The model under review builds one solid part; all positions refer to its coordinate system, in mm. A direction names the side the tool comes from. Coordinates: 2 decimals unless noted, no trailing zeros. Write each loop counter-clockwise with the first axis right and the second up, starting at its lowest first coordinate (ties: lowest second). Pieces come first, ordered by that corner, then holes.
Autodesk Inventor part; units mm, degrees
ref_plane "YZ Plane" through (0, 0, 0) normal (1, 0, 0) x (0, 1, 0)
ref_plane "XZ Plane" through (0, 0, 0) normal (0, 1, 0) x (-1, 0, 0)
ref_plane "XY Plane" through (0, 0, 0) normal (0, 0, 1) x (1, 0, 0)
sketch "Sketch1" plane through (0, 0, 0) normal (0, 0, 1) x (1, 0, 0)
  arc A0 (8.5146, 0.7768) -> (-8.5146, 0.7768) centre (0, 0) ccw
  line L0 (-18.6378, -8.55) -> (-30, -8.55)
  line L1 (30, -8.55) -> (30, -5.55)
  line L2 (30, -5.55) -> (17.1, -5.55)
  line L3 (-30, -8.55) -> (-30, -5.55)
  line L4 (-30, -5.55) -> (-17.1, -5.55)
  arc A1 (11.55, 0) -> (17.1, -5.55) centre (19.2544, 2.1544) ccw
  line L5 (11.55, 0) -> (17.1, -5.55) construction
  line L6 (11.55, 0) -> (19.3989, 0) construction
  arc A2 (8.4438, 1.3433) -> (18.6378, -8.55) centre (19.3906, 2.4242) ccw
  arc A3 (-17.1, -5.55) -> (-11.55, 0) centre (-19.2544, 2.1544) ccw
  arc A4 (-18.6378, -8.55) -> (-8.4438, 1.3433) centre (-19.3906, 2.4242) ccw
  line L7 (18.6378, -8.55) -> (30, -8.55)
  arc A5 (11.55, 0) -> (-11.55, 0) centre (0, 0) ccw
  dimension "d0" = 17.1
  dimension "d3" = 3
  dimension "d6" = 45
  dimension "d7" = 8
  dimension "d8" = 11
extrude "Extrusion1" add sketch "Sketch1" against normal blind 10 contours A0 A4 L0 L3 L4 A3 A5 A1 L2 L1 L7 A2
sketch "Sketch2" plane through (17.1, -5.55, 0) normal (0, 1, 0) x (1, 0, 0)
  circle A0 centre (6.45, 5) radius 1.5
  point P0 (-17.1, 0)
  dimension "d11" = 3
hole "Hole1" at (23.55, -5.55, -5) direction (0, -1, 0) diameter 3 end through all
sketch "Sketch3" plane through (-30, -5.55, 0) normal (0, 1, 0) x (1, 0, 0)
  circle A0 centre (6.45, 5) radius 1.5
  point P0 (30, 0)
  dimension "d19" = 3
hole "Hole2" at (-23.55, -5.55, -5) direction (0, -1, 0) diameter 3 end through all
sketch "Sketch4" plane through (-30, -8.55, 0) normal (0, -1, 0) x (1, 0, 0)
  circle A0 centre (6.45, -5) radius 1.5
  line L0 (0, -10) -> (11.3622, -10)
  line L1 (11.3622, 0) -> (11.3622, -10)
  line L2 (0, 0) -> (11.3622, 0)
  line L3 (0, 0) -> (0, -10)
  point P0 (30, 0)
properties part number "braket motor kipas"
Item 1: Take a section at A-A, the plane y = -4.75. Write out the cut boundary in (x, z).
Solved:
outline: (-15.21, -10) - (-11.05, -10) - (-11.05, 0) - (-15.21, 0) - close; (11.05, -10) - (15.21, -10) - (15.21, 0) - (11.05, 0) - close
Item 2: Take a section at B-B, the plane x = 23.55. Write out the cut boundary in (y, z), plus the area to 3 significant figures.
Solved:
outline: (-8.55, -10) - (-5.55, -10) - (-5.55, -6.5) - (-8.55, -6.5) - close; (-8.55, -3.5) - (-5.55, -3.5) - (-5.55, 0) - (-8.55, 0) - close
area: 21.0 mm2
Item 3: Take a section at D-D, the plane z = -5. Write out the cut boundary in (x, y), plus the area to 3 significant figures.
Solved:
outline: (-30, -8.55) - (-25.05, -8.55) - (-25.05, -5.55) - (-30, -5.55) - close; (-22.05, -8.55) - (-18.64, -8.55) arc R11 ccw to (-8.51, 0.78) arc R8.55 cw to (8.51, 0.78) arc R11 ccw to (18.64, -8.55) - (22.05, -8.55) - (22.05, -5.55) - (17.1, -5.55) arc R8 cw to (11.55, 0) arc R11.55 ccw to (-11.55, 0) arc R8 cw to (-17.1, -5.55) - (-22.05, -5.55) - close; (25.05, -8.55) - (30, -8.55) - (30, -5.55) - (25.05, -5.55) - close
area: 210 mm2
Item 4: Mouldability with a two-part tool opening along X and no side actions: class faces 4 (the face through (0.254, 11.547, -4.93)), 5 (the face through (25, -5.55, -4)), 6 (the face through (11.861, -5.595, -4.93)) as pulls with the +X half, pulls with the -X half, needs draft (parallel to the pull), parting line crosses it, or undercut.
Solved:
face 4: parting line crosses it
face 5: needs draft
face 6: undercut
Item 5: Machinability: for faces 1 (the face through (-12.014, -5.736, -4.93)), 2 (the face through (-22.086, -7.071, -5.325)), 3 (the face through (-25, -5.55, -4)), which of the approach directions +Z, -Z, +X, -X, +Y, -Y give a long, thin tool a straight path to every point of the face, cutting with its end or side? Answer none if there is none.
Solved:
face 1: +Z, -Z, -Y
face 2: +Y, -Y
face 3: +Z, -Z, -X, +Y
Item 6: To check wall thickness, follow line 1 along Z through (x, y) = (-23.55, -7.55); line 2 along X through (y, z) = (-7.6, -5); line 3 along Y through (x, z) = (27, -0.5). State the ranges of each line that lie inside material, in increasing order.
Solved:
line 1: z = -10 to -6.5, -3.5 to 0
line 2: x = -30 to -25.05, -22.05 to -14.86, 14.86 to 22.05, 25.05 to 30
line 3: y = -8.55 to -5.55
Item 7: Take a section at C-C, the plane z = -1. Write out the cut boundary in (x, y), plus the area to 3 significant figures.
Solved:
outline: (-30, -8.55) - (-18.64, -8.55) arc R11 ccw to (-8.51, 0.78) arc R8.55 cw to (8.51, 0.78) arc R11 ccw to (18.64, -8.55) - (30, -8.55) - (30, -5.55) - (17.1, -5.55) arc R8 cw to (11.55, 0) arc R11.55 ccw to (-11.55, 0) arc R8 cw to (-17.1, -5.55) - (-30, -5.55) - close
area: 228 mm2
Item 8: For pin 1 (2 mm diameter, centred on x = 7, z = -1, fed in from +Y); pin 2 (4 mm diameter, centred on y = -3, z = -5, fed in from +X); pin 3 (5 mm diameter, centred on x = 22, z = -5.5, fed in from +Y); pin 4 (5 mm diameter, centred on x = 23.55, z = -5, fed in from -Y), all flat-tipped, find the tip position at first contact; note any pin that passes through.
Solved:
pin 1: stops at y = 9.87
pin 2: stops at x = 15.67
pin 3: stops at y = -5.55
pin 4: stops at y = -8.55
